```python
from build123d import *

# Parameters (mm, degrees)
BOSS_EXTRU_1_DEPTH      = 40
ENL_V_MAT_EXTRU_1_REACH = 322.156
ESQUISSE2_R             = 9.5
ESQUISSE2_R_2           = 7.75
ESQUISSE2_R_3           = 6.5


with BuildPart() as part:
    # Esquisse1 → Boss.-Extru.1 (new body)
    with BuildSketch(Plane.XY):
        with BuildLine():
            Line((-74.833147735, 130), (74.833147735, 130))
            ThreePointArc((74.833147735, 130), (0, -150), (-74.833147735, 130))
        make_face()
        with BuildLine():
            Line((-74.296702484, 128), (74.296702484, 128))
            ThreePointArc((74.296702484, 128), (0, -148), (-74.296702484, 128))
        make_face(mode=Mode.SUBTRACT)
    extrude(amount=BOSS_EXTRU_1_DEPTH)

    # Esquisse2 → Enlèv. mat.-Extru.1 (cut, up to next)
    with BuildSketch(Plane(origin=(0, 130, 0), x_dir=(1, 0, 0), z_dir=(0, 1, 0)), mode=Mode.PRIVATE) as enl_v_mat_extru_1_sk1:
        with Locations(Location((60, -20, 0), (0, 0, 270))):
            Circle(ESQUISSE2_R)
    enl_v_mat_extru_1_tool1 = extrude(enl_v_mat_extru_1_sk1.sketch, amount=-ENL_V_MAT_EXTRU_1_REACH, mode=Mode.PRIVATE) & part.part
    # Esquisse2 → Enlèv. mat.-Extru.1 (cut, up to next)
    with BuildSketch(Plane(origin=(0, 130, 0), x_dir=(1, 0, 0), z_dir=(0, 1, 0)), mode=Mode.PRIVATE) as enl_v_mat_extru_1_sk2:
        with Locations(Location((-60, -20, 0), (0, 0, 270))):
            Circle(ESQUISSE2_R_2)
    enl_v_mat_extru_1_tool2 = extrude(enl_v_mat_extru_1_sk2.sketch, amount=-ENL_V_MAT_EXTRU_1_REACH, mode=Mode.PRIVATE) & part.part
    # Esquisse2 → Enlèv. mat.-Extru.1 (cut, up to next)
    with BuildSketch(Plane(origin=(0, 130, 0), x_dir=(1, 0, 0), z_dir=(0, 1, 0)), mode=Mode.PRIVATE) as enl_v_mat_extru_1_sk3:
        with Locations(Location((30, -20, 0), (0, 0, 270))):
            Circle(ESQUISSE2_R_3)
    enl_v_mat_extru_1_tool3 = extrude(enl_v_mat_extru_1_sk3.sketch, amount=-ENL_V_MAT_EXTRU_1_REACH, mode=Mode.PRIVATE) & part.part
    add(enl_v_mat_extru_1_tool1.solids().sort_by_distance((60, 130, 20))[0], mode=Mode.SUBTRACT)
    add(enl_v_mat_extru_1_tool2.solids().sort_by_distance((-60, 130, 20))[0], mode=Mode.SUBTRACT)
    add(enl_v_mat_extru_1_tool3.solids().sort_by_distance((30, 130, 20))[0], mode=Mode.SUBTRACT)


solid = part.part
```
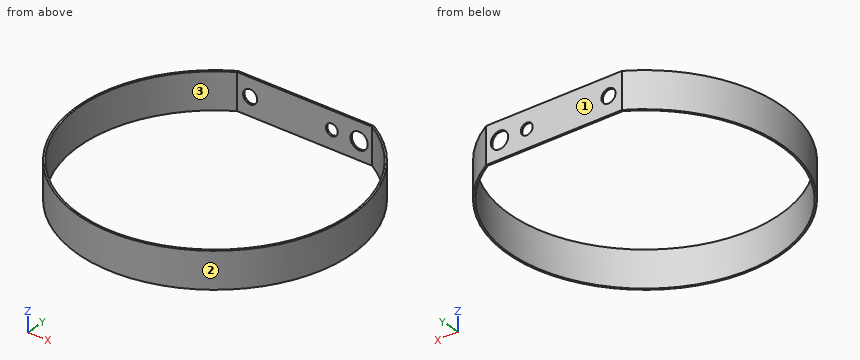
Here's how the part is built. I have some questions about the finished solid (model axes, mm). Face numbers are marked on the shaded views. Round coordinates to 2 decimals unless told otherwise and drop trailing zeros. Order: outer loops, then holes, each group sorted by start corner. A loop starts at its lowest first (then second) coordinate and runs counter-clockwise, first axis right, second up. Notation, with made-up numbers: M 9.5,73.25 L 34.5,73.25 A16 ccw 34.5,98.25 Z; hole C 64.5,-25.5 d6. An arc over 180 degrees is marked long. Answer in a Markdown table with one row per item.
Item 1: Imagine slicing it at D-D, the plane x = 60. Write out the boundary of the cut face in (y, z).
A:
| item | result |
|---|---|
| outline | M -137.48,0 L -135.29,0 L -135.29,40 L -137.48,40 Z; M 128,0 L 130,0 L 130,10.5 L 128,10.5 Z; M 128,29.5 L 130,29.5 L 130,40 L 128,40 Z |
Item 2: Imagine slicing it at B-B, the plane z = 20. Write out the boundary of the cut face in (x, y), and give its area (3 significant figures).
A:
| item | result |
|---|---|
| outline | M -74.83,130 A150 ccw long 74.83,130 L 69.5,130 L 69.5,128 L 74.3,128 A148 cw long -74.3,128 L -67.75,128 L -67.75,130 Z; M -52.25,128 L 23.5,128 L 23.5,130 L -52.25,130 Z; M 36.5,128 L 50.5,128 L 50.5,130 L 36.5,130 Z |
| area | 1,760 mm2 |
Item 3: Imagine slicing it at A-A, the plane y = 0. Write out the boundary of the cut face in (x, z).
A:
| item | result |
|---|---|
| outline | M -150,0 L -148,0 L -148,40 L -150,40 Z; M 148,0 L 150,0 L 150,40 L 148,40 Z |
Item 4: I'm going to push flat-ended pins straight in: pin 1 (2 mm diameter, centred on x = -17, z = 35.5, fed in from -Y); pin 2 (12 mm diameter, centred on y = -61.5, z = 9.5, fed in from +X); pin 3 (18 mm diameter, centred on x = -60, z = 20, fed in from +Y); pin 4 (3 mm diameter, centred on x = -58, z = 15, fed in from -Y). Where does each tip first touch, or does it pass through?
A:
| item | result |
|---|---|
| pin 1 | stops at y = -149.14 |
| pin 2 | stops at x = 139.35 |
| pin 3 | stops at y = 130 |
| pin 4 | stops at y = -138.95 |
Item 5: Thinking about a two-plate mould opening in X: for the marked faces 1, 2 and 3, which applies, +X half, -X half, draft (parallel to the pull), parting line (faces both ways), or undercut?
A:
| item | result |
|---|---|
| face 1 | draft |
| face 2 | parting line |
| face 3 | undercut |
Item 6: If I drill on L1, parallel to X at y = 0, z = 17; L2, parallel to X at y = 129, z = 20; L3, parallel to Y at x = 0, z = 28, over which ranges is the centre line in solid material (lowest first)? Write a range as from..to.
A:
| item | result |
|---|---|
| L1 | x = -150..-148, 148..150 |
| L2 | x = -76.54..-67.75, -52.25..23.5, 36.5..50.5, 69.5..76.54 |
| L3 | y = -150..-148, 128..130 |
Item 7: Imagine slicing it at C-C, the plane x = 0. Write out the boundary of the cut face in (y, z), and give its area (3 significant figures).
A:
| item | result |
|---|---|
| outline | M -150,0 L -148,0 L -148,40 L -150,40 Z; M 128,0 L 130,0 L 130,40 L 128,40 Z |
| area | 160 mm2 |
